```python
from build123d import *

# Parameters (mm, degrees)
F0_W     = 30.48
F0_H     = 33.528
F0_W_2   = 1.778
F0_H_2   = 2.7663977579
F0_H_3   = 1.9106194377
F0_H_4   = 3.7477533333
F0_H_5   = 3.6007831804
F0_H_6   = 2.099653706
F0_H_7   = 2.7503813617
F0_H_8   = 3.4538120963
F0_H_9   = 3.9107408137
F0_W_3   = 3.1533570525
F0_W_4   = 3.2304820977
F0_W_5   = 2.6331608498
F0_W_6   = 3.0382862671
F0_W_7   = 3.5224076404
F0_W_8   = 2.4563060925
F1_DEPTH = 3.048
F2_SIZE  = 1.27


with BuildPart() as f1:
    # F0 (on Front) → F1 (new body)
    with BuildSketch(Plane.XZ):
        Rectangle(F0_W, F0_H)
        Polygon((-13.462, 12.2196022421), (-13.462, 14.986), (-11.0056939075, 14.986), (-9.2276939075, 14.986), (-5.7052862671, 14.986), (-3.9272862671, 14.986), (-0.889, 14.986), (0.889, 14.986), (3.5221608498, 14.986), (5.3001608498, 14.986), (8.5306429475, 14.986), (10.3086429475, 14.986), (13.462, 14.986), (13.462, 12.2196022421), (13.462, 10.3089828044), (13.462, 6.5612294711), (13.462, 4.6506100334), (13.462, 1.049826853), (13.462, -1.049826853), (13.462, -3.8002082147), (13.462, -5.7108276524), (13.462, -9.1646397486), (13.462, -11.0752591863), (13.462, -14.986), (10.3086429475, -14.986), (8.5306429475, -14.986), (5.3001608498, -14.986), (3.5221608498, -14.986), (0.889, -14.986), (-0.889, -14.986), (-3.9272862671, -14.986), (-5.7052862671, -14.986), (-9.2276939075, -14.986), (-11.0056939075, -14.986), (-13.462, -14.986), (-13.462, -11.0752591863), (-13.462, -9.1646397486), (-13.462, -5.7108276524), (-13.462, -3.8002082147), (-13.462, -1.049826853), (-13.462, 1.049826853), (-13.462, 4.6506100334), (-13.462, 6.5612294711), (-13.462, 10.3089828044), align=None, mode=Mode.SUBTRACT)
        with Locations((-10.1166939075, 13.6028011211)):
            Rectangle(F0_W_2, F0_H_2)
        with Locations((-10.1166939075, 11.2642925233)):
            Rectangle(F0_W_2, F0_H_3)
        with Locations((-10.1166939075, 8.4351061378)):
            Rectangle(F0_W_2, F0_H_4)
        with Locations((-10.1166939075, 5.6059197523)):
            Rectangle(F0_W_2, F0_H_3)
        with Locations((-10.1166939075, 2.8502184432)):
            Rectangle(F0_W_2, F0_H_5)
        with Locations((-10.1166939075, 0)):
            Rectangle(F0_W_2, F0_H_6)
        with Locations((-10.1166939075, -2.4250175338)):
            Rectangle(F0_W_2, F0_H_7)
        with Locations((-10.1166939075, -4.7555179335)):
            Rectangle(F0_W_2, F0_H_3)
        with Locations((-10.1166939075, -7.4377337005)):
            Rectangle(F0_W_2, F0_H_8)
        with Locations((-10.1166939075, -10.1199494675)):
            Rectangle(F0_W_2, F0_H_3)
        with Locations((-10.1166939075, -13.0306295932)):
            Rectangle(F0_W_2, F0_H_9)
        with Locations((-4.8162862671, -13.0306295932)):
            Rectangle(F0_W_2, F0_H_9)
        with Locations((-4.8162862671, -10.1199494675)):
            Rectangle(F0_W_2, F0_H_3)
        with Locations((-4.8162862671, -7.4377337005)):
            Rectangle(F0_W_2, F0_H_8)
        with Locations((-4.8162862671, -4.7555179335)):
            Rectangle(F0_W_2, F0_H_3)
        with Locations((-4.8162862671, -2.4250175338)):
            Rectangle(F0_W_2, F0_H_7)
        with Locations((-4.8162862671, 0)):
            Rectangle(F0_W_2, F0_H_6)
        with Locations((-4.8162862671, 2.8502184432)):
            Rectangle(F0_W_2, F0_H_5)
        with Locations((-4.8162862671, 5.6059197523)):
            Rectangle(F0_W_2, F0_H_3)
        with Locations((-4.8162862671, 8.4351061378)):
            Rectangle(F0_W_2, F0_H_4)
        with Locations((-4.8162862671, 11.2642925233)):
            Rectangle(F0_W_2, F0_H_3)
        with Locations((-4.8162862671, 13.6028011211)):
            Rectangle(F0_W_2, F0_H_2)
        with Locations((0, 13.6028011211)):
            Rectangle(F0_W_2, F0_H_2)
        with Locations((0, 11.2642925233)):
            Rectangle(F0_W_2, F0_H_3)
        with Locations((0, 8.4351061378)):
            Rectangle(F0_W_2, F0_H_4)
        with Locations((0, 5.6059197523)):
            Rectangle(F0_W_2, F0_H_3)
        with Locations((0, 2.8502184432)):
            Rectangle(F0_W_2, F0_H_5)
        Rectangle(F0_W_2, F0_H_6)
        with Locations((0, -2.4250175338)):
            Rectangle(F0_W_2, F0_H_7)
        with Locations((0, -4.7555179335)):
            Rectangle(F0_W_2, F0_H_3)
        with Locations((0, -7.4377337005)):
            Rectangle(F0_W_2, F0_H_8)
        with Locations((0, -10.1199494675)):
            Rectangle(F0_W_2, F0_H_3)
        with Locations((0, -13.0306295932)):
            Rectangle(F0_W_2, F0_H_9)
        with Locations((4.4111608498, -13.0306295932)):
            Rectangle(F0_W_2, F0_H_9)
        with Locations((4.4111608498, -10.1199494675)):
            Rectangle(F0_W_2, F0_H_3)
        with Locations((4.4111608498, -7.4377337005)):
            Rectangle(F0_W_2, F0_H_8)
        with Locations((4.4111608498, -4.7555179335)):
            Rectangle(F0_W_2, F0_H_3)
        with Locations((4.4111608498, -2.4250175338)):
            Rectangle(F0_W_2, F0_H_7)
        with Locations((4.4111608498, 0)):
            Rectangle(F0_W_2, F0_H_6)
        with Locations((4.4111608498, 2.8502184432)):
            Rectangle(F0_W_2, F0_H_5)
        with Locations((4.4111608498, 5.6059197523)):
            Rectangle(F0_W_2, F0_H_3)
        with Locations((4.4111608498, 8.4351061378)):
            Rectangle(F0_W_2, F0_H_4)
        with Locations((4.4111608498, 11.2642925233)):
            Rectangle(F0_W_2, F0_H_3)
        with Locations((4.4111608498, 13.6028011211)):
            Rectangle(F0_W_2, F0_H_2)
        with Locations((9.4196429475, 13.6028011211)):
            Rectangle(F0_W_2, F0_H_2)
        with Locations((9.4196429475, 11.2642925233)):
            Rectangle(F0_W_2, F0_H_3)
        with Locations((9.4196429475, 8.4351061378)):
            Rectangle(F0_W_2, F0_H_4)
        with Locations((9.4196429475, 5.6059197523)):
            Rectangle(F0_W_2, F0_H_3)
        with Locations((9.4196429475, 2.8502184432)):
            Rectangle(F0_W_2, F0_H_5)
        with Locations((9.4196429475, 0)):
            Rectangle(F0_W_2, F0_H_6)
        with Locations((9.4196429475, -2.4250175338)):
            Rectangle(F0_W_2, F0_H_7)
        with Locations((9.4196429475, -4.7555179335)):
            Rectangle(F0_W_2, F0_H_3)
        with Locations((9.4196429475, -7.4377337005)):
            Rectangle(F0_W_2, F0_H_8)
        with Locations((9.4196429475, -10.1199494675)):
            Rectangle(F0_W_2, F0_H_3)
        with Locations((9.4196429475, -13.0306295932)):
            Rectangle(F0_W_2, F0_H_9)
        with Locations((11.8853214738, -10.1199494675)):
            Rectangle(F0_W_3, F0_H_3)
        with Locations((6.9154018987, -10.1199494675)):
            Rectangle(F0_W_4, F0_H_3)
        with Locations((2.2055804249, -10.1199494675)):
            Rectangle(F0_W_5, F0_H_3)
        with Locations((-2.4081431336, -10.1199494675)):
            Rectangle(F0_W_6, F0_H_3)
        with Locations((-7.4664900873, -10.1199494675)):
            Rectangle(F0_W_7, F0_H_3)
        with Locations((-12.2338469538, -10.1199494675)):
            Rectangle(F0_W_8, F0_H_3)
        with Locations((-12.2338469538, -4.7555179335)):
            Rectangle(F0_W_8, F0_H_3)
        with Locations((-7.4664900873, -4.7555179335)):
            Rectangle(F0_W_7, F0_H_3)
        with Locations((-2.4081431336, -4.7555179335)):
            Rectangle(F0_W_6, F0_H_3)
        with Locations((2.2055804249, -4.7555179335)):
            Rectangle(F0_W_5, F0_H_3)
        with Locations((6.9154018987, -4.7555179335)):
            Rectangle(F0_W_4, F0_H_3)
        with Locations((11.8853214738, -4.7555179335)):
            Rectangle(F0_W_3, F0_H_3)
        with Locations((11.8853214738, 0)):
            Rectangle(F0_W_3, F0_H_6)
        with Locations((6.9154018987, 0)):
            Rectangle(F0_W_4, F0_H_6)
        with Locations((2.2055804249, 0)):
            Rectangle(F0_W_5, F0_H_6)
        with Locations((-2.4081431336, 0)):
            Rectangle(F0_W_6, F0_H_6)
        with Locations((-7.4664900873, 0)):
            Rectangle(F0_W_7, F0_H_6)
        with Locations((-12.2338469538, 0)):
            Rectangle(F0_W_8, F0_H_6)
        with Locations((-12.2338469538, 5.6059197523)):
            Rectangle(F0_W_8, F0_H_3)
        with Locations((-7.4664900873, 5.6059197523)):
            Rectangle(F0_W_7, F0_H_3)
        with Locations((-2.4081431336, 5.6059197523)):
            Rectangle(F0_W_6, F0_H_3)
        with Locations((2.2055804249, 5.6059197523)):
            Rectangle(F0_W_5, F0_H_3)
        with Locations((6.9154018987, 5.6059197523)):
            Rectangle(F0_W_4, F0_H_3)
        with Locations((11.8853214738, 5.6059197523)):
            Rectangle(F0_W_3, F0_H_3)
        with Locations((11.8853214738, 11.2642925233)):
            Rectangle(F0_W_3, F0_H_3)
        with Locations((6.9154018987, 11.2642925233)):
            Rectangle(F0_W_4, F0_H_3)
        with Locations((2.2055804249, 11.2642925233)):
            Rectangle(F0_W_5, F0_H_3)
        with Locations((-2.4081431336, 11.2642925233)):
            Rectangle(F0_W_6, F0_H_3)
        with Locations((-7.4664900873, 11.2642925233)):
            Rectangle(F0_W_7, F0_H_3)
        with Locations((-12.2338469538, 11.2642925233)):
            Rectangle(F0_W_8, F0_H_3)
    extrude(amount=F1_DEPTH)

    # F2
    f2_edges = [f1.edges().sort_by_distance(p)[0] for p in [
        (-15.24, -3.048, 0),
        (0, -3.048, -16.764),
        (15.24, -3.048, 0),
        (0, -3.048, 16.764),
    ]]
    chamfer(f2_edges, length=F2_SIZE)


solid = f1.part
```
Verification items for the finished model (mm, model axes). A direction names the side the tool comes from. Give positions to 0.01 mm unless a question says otherwise; leave off trailing zeros. Answer in a Markdown table with one row per item. Add a question column.
Item 1: Tool access check on faces 1 (the flat face through (7, -2, 14.986)), 2 (the flat face through (-0.21, -2.42, 16.12)). Record the directions out of +Z, -Z, +X, -X, +Y, -Y that give a thin tool (end or side, any length) a straight path to the whole face; none if there is none.
Item 2: Scan lines: probe 1 along Z at (x, y) = (-4, -2.3); probe 2 along Y at (x, z) = (-14, -6); probe 3 along Z at (x, y) = (4, -2.5). Record each from-to range of solid material in increasing order. Write a range as from..to.
Item 3: Gauge pin test, flat end, axial feed: pin 1 (1 mm diameter, centred on x = 4.5, y = -2.5, fed in from +Z). Record the tip position at first contact, or that the pin passes through.
Item 4: Section check A-A, the plane x = -13. State how many separate pieces and enclosed holes the cut face has, and give its area (3 significant figures).
Item 5: Mould release check, pull along Z, two halves, no side actions. Record for faces 3 (the flat face through (12, -2, 6.561)), 4 (the flat face through (0, -1, 16.764)): released by +Z, released by -Z, zero draft, split by the parting line, or undercut.
Filled sheet:
| question | item | result |
|---|---|---|
| 1 | face 1 | +Y, -Y |
| 1 | face 2 | +Z, +X, -X, -Y |
| 2 | probe 1 | z = -16.24..16.24 |
| 2 | probe 2 | y = -3.02..0 |
| 2 | probe 3 | z = -16.04..16.04 |
| 3 | pin 1 | stops at z = 16.54 |
| 4 | separate pieces | 7 |
| 4 | enclosed holes | 0 |
| 4 | area | 38.9 mm^2 |
| 5 | face 3 | undercut |
| 5 | face 4 | released by +Z |
